```python
from build123d import *

# Parameters (mm, degrees)
SKETCH1_R           = 1.6
BOSS_EXTRUDE1_DEPTH = 1.5
FILLET1_R           = 5
CUT_EXTRUDE1_DEPTH  = 1.5
SKETCH3_R           = 1.6
CUT_EXTRUDE2_DEPTH  = 1.5
SKETCH4_R           = 3
SKETCH4_R_2         = 1.6
BOSS_EXTRUDE2_DEPTH = 1.5
SKETCH5_R           = 3
CUT_EXTRUDE3_DEPTH  = 1


with BuildPart() as part:
    # Sketch1 → Boss-Extrude1 (new body)
    with BuildSketch(Plane.XY):
        with BuildLine():
            Line((32.770526581, 29), (-0.138438763, 48))
            ThreePointArc((-0.138438763, 48), (-13, 0), (-0.138438763, -48))
            Line((-0.138438763, -48), (32.770526581, -29))
            ThreePointArc((32.770526581, -29), (25, 0), (32.770526581, 29))
        make_face()
        with Locations((0, 15)):
            Circle(SKETCH1_R, mode=Mode.SUBTRACT)
        with Locations((15, 15)):
            Circle(SKETCH1_R, mode=Mode.SUBTRACT)
        with Locations((15, -15)):
            Circle(SKETCH1_R, mode=Mode.SUBTRACT)
        with Locations((0, -15)):
            Circle(SKETCH1_R, mode=Mode.SUBTRACT)
    extrude(amount=BOSS_EXTRUDE1_DEPTH)

    # Fillet1
    fillet1_edges = [part.edges().sort_by_distance(p)[0] for p in [
        (32.770526581, -29, 0.75),
        (-0.138438763, -48, 0.75),
        (-0.138438763, 48, 0.75),
        (32.770526581, 29, 0.75),
    ]]
    fillet(fillet1_edges, radius=FILLET1_R)

    # Sketch2 → Cut-Extrude1 (cut)
    with BuildSketch(Plane.XY.offset(1.5)):
        Polygon((83, 0), (-2.650210769, 43.359444129), (-7.007085146, 61.211012317), (87.93666147, 66.514409607), (145.627275899, 17.878375919), (122.602770589, -61.543232286), (-16.449719346, -74.090294168), (-2.650210769, -43.359444129), align=None)
    extrude(amount=-CUT_EXTRUDE1_DEPTH, mode=Mode.SUBTRACT)

    # Sketch3 → Cut-Extrude2 (cut)
    with BuildSketch(Plane.XY.offset(1.5)):
        with Locations((6.279196304, 38.839033454)):
            Circle(SKETCH3_R)
        with Locations((-7.270629986, 12.073342588)):
            Circle(SKETCH3_R)
        with Locations((24.848199053, -4.18644896)):
            Circle(SKETCH3_R)
    extrude(amount=-CUT_EXTRUDE2_DEPTH, mode=Mode.SUBTRACT)

    # Sketch4 → Boss-Extrude2 (add)
    with BuildSketch(Plane.XY.offset(1.5)):
        with Locations((6.279196304, 38.839033454)):
            Circle(SKETCH4_R)
        with Locations((6.279196304, 38.839033454)):
            Circle(SKETCH4_R_2, mode=Mode.SUBTRACT)
        with Locations((24.848199053, -4.18644896)):
            Circle(SKETCH4_R)
        with Locations((24.848199053, -4.18644896)):
            Circle(SKETCH4_R_2, mode=Mode.SUBTRACT)
    extrude(amount=-BOSS_EXTRUDE2_DEPTH)

    # Sketch5 → Cut-Extrude3 (cut)
    with BuildSketch(Plane.XY.offset(1.5)):
        with Locations((0, 15)):
            Circle(SKETCH5_R)
        with Locations((15, 15)):
            Circle(SKETCH5_R)
        with Locations((15, -15)):
            Circle(SKETCH5_R)
        with Locations((0, -15)):
            Circle(SKETCH5_R)
    extrude(amount=-CUT_EXTRUDE3_DEPTH, mode=Mode.SUBTRACT)


solid = part.part
```
Can you work these out from the model? Positions are in its coordinate system, mm. A direction names the side the tool comes from. Give positions to 0.01 mm unless a question says otherwise; leave off trailing zeros. Loops run counter-clockwise (first coordinate to the right, second up) from the corner with the lowest first, then second, coordinate; pieces in that order, holes last. Notation, with made-up numbers: M 82,-3.5 L 140,-3.5 A23 ccw 140,16.5 Z; hole C 60,75 d1. An arc over 180 degrees is marked long. Answer in a Markdown table with one row per item.
1. Thinking about a two-plate mould opening in Y: for faces 1 (the flat face through (9, 1, 0)), 2 (the cylindrical face through (-0.208, 16.586, 0.246)), 3 (the flat face through (0.52, 41.755, 0.76)), which applies, released by +Y, released by -Y, zero draft, split by the parting line, or undercut?
Taken from the geometry:
| item | result |
|---|---|
| face 1 | zero draft |
| face 2 | undercut |
| face 3 | released by +Y |
2. If I drill on line 1 along Y through (x, z) = (15.5, 0.4); line 2 along Y through (x, z) = (0, 1.1); line 3 along X through (y, z) = (-15.5, 1.1), over which ranges is the centre line in solid material (lowest first)?
Taken from the geometry:
| item | result |
|---|---|
| line 1 | y = -34.17 to -16.52, -13.48 to 13.48, 16.52 to 34.17 |
| line 2 | y = -42.02 to -18, -12 to 12, 18 to 42.02 |
| line 3 | x = -11.74 to -2.96, 2.96 to 12.04, 17.96 to 27.11 |
3. Which directions (+Z, -Z, +X, -X, +Y, -Y) give clear straight access to the entire face, cutting with the end or side of a thin tool? Please do faces 4 (the cylindrical face through (-5.745, 12.554, 0.76)), 5 (the cylindrical face through (27.355, -16.358, 0.74)), 6 (the flat face through (16.3, -16.3, 0.5)).
Taken from the geometry:
| item | result |
|---|---|
| face 4 | +Z, -Z |
| face 5 | +Z, -Z, +X |
| face 6 | +Z |
4. For pin 1 Ø9.5 at (x, y) = (0, -15) entering from -Z; pin 2 Ø3 at (x, y) = (14.5, 14.5) entering from +Z; pin 3 Ø2.5 at (x, y) = (6.28, 38.84) entering from +Z, each with a flat end and sliding along its axis, tell me the tip position at first contact or that it passes through.
Taken from the geometry:
| item | result |
|---|---|
| pin 1 | stops at z = 0 |
| pin 2 | stops at z = 0.5 |
| pin 3 | passes through |
5. Suppose I cut it at C-C on z = 0.8. Write out the boundary of the cut face in (x, y).
Taken from the geometry:
| item | result |
|---|---|
| outline | M -2.65,-43.36 L 31.05,-26.3 A5 ccw 30.63,-24.92 A58 cw 25.44,-7.13 A3 ccw 25.01,-1.19 A58 cw 30.63,24.92 A5 ccw 31.05,26.3 L 8.96,37.48 A3 ccw 3.6,40.19 L -2.65,43.36 A96 ccw Z; hole C -7.27,12.07 d3.2; hole C 0,-15 d6; hole C 0,15 d6; hole C 6.28,38.84 d3.2; hole C 15,-15 d6; hole C 15,15 d6; hole C 24.85,-4.19 d3.2 |
6. Suppose I cut it at A-A on y = -15. Write out the boundary of the cut face in (x, z), plus the area to 3 significant figures.
Taken from the geometry:
| item | result |
|---|---|
| outline | M -11.82,0 L -1.6,0 L -1.6,0.5 L -3,0.5 L -3,1.5 L -11.82,1.5 Z; M 1.6,0 L 13.4,0 L 13.4,0.5 L 12,0.5 L 12,1.5 L 3,1.5 L 3,0.5 L 1.6,0.5 Z; M 16.6,0 L 26.97,0 L 26.97,1.5 L 18,1.5 L 18,0.5 L 16.6,0.5 Z |
| area | 43.0 mm² |
7. Suppose I cut it at D-D on x = 22. Write out the boundary of the cut face in (y, z).
Taken from the geometry:
| item | result |
|---|---|
| outline | M -30.88,0 L 30.88,0 L 30.88,1.5 L -30.88,1.5 Z |
8. Suppose I cut it at B-B on x = 15. Write out the boundary of the cut face in (y, z).
Taken from the geometry:
| item | result |
|---|---|
| outline | M -34.42,0 L -16.6,0 L -16.6,0.5 L -18,0.5 L -18,1.5 L -34.42,1.5 Z; M -13.4,0 L 13.4,0 L 13.4,0.5 L 12,0.5 L 12,1.5 L -12,1.5 L -12,0.5 L -13.4,0.5 Z; M 16.6,0 L 34.42,0 L 34.42,1.5 L 18,1.5 L 18,0.5 L 16.6,0.5 Z |
